Geometry check sheet. Reference: the model listing, model coordinates, mm. A direction names the side the tool comes from. Round coordinates to 2 decimals unless told otherwise and drop trailing zeros. Order: outer loops, then holes, each group sorted by start corner. A loop starts at its lowest first (then second) coordinate and runs counter-clockwise, first axis right, second up.
(1) Cross-section at B-B on x = 1.3. Count the separate pieces of the cut face and the enclosed holes in it, and give its area (3 significant figures).
(2) Cross-section at A-A on y = 105.5. Enter the section's corners in (x, z), and give its area (3 significant figures).
(3) Thickness scan on L1, parallel to Y at x = 0.95, z = 73.5; L2, parallel to Y at x = 1.4, z = 54; L3, parallel to Z at x = 0.15, y = -62.5. Record the ranges inside material, lowest first.
(4) Draft check along Y on faces 3 (the face through (0.811, -92.508, 55.896)), 4 (the face through (0.811, 154.312, 24.605)), 5 (the face through (0.789, 158.651, 69.018)). Enter one of: pulls with the +Y half, pulls with the -Y half, needs draft (parallel to the pull), parting line crosses it, or undercut.
(5) Cross-section at C-C on y = 177.5. Enter the section's corners in (x, z).
(6) Set-up check for faces 1 (the face through (1.6, 16, 38)), 2 (the face through (0.81, 139.3, 51.42)): record each of +Z, -Z, +X, -X, +Y, -Y from which the full face is reachable in a straight line by a thin tool's end or side.
(7) Gauge pin test, flat end, axial feed: P1, Ø3.5, axis at y = 189.88, z = 74, coming from the -X side. Record the tip position at first contact, or that the pin passes through.
Autodesk Inventor part; units mm, degrees
ref_plane "YZ Plane" through (0, 0, 0) normal (1, 0, 0) x (0, 1, 0)
ref_plane "XZ Plane" through (0, 0, 0) normal (0, 1, 0) x (-1, 0, 0)
ref_plane "XY Plane" through (0, 0, 0) normal (0, 0, 1) x (1, 0, 0)
sketch "Esquisse1" plane through (0, 0, 0) normal (1, 0, 0) x (0, 1, 0)
  line L0 (-80, -0.3825) -> (90, -0.3825)
  line L1 (90, -0.3825) -> (155.7273, 23)
  line L2 (155.7273, 23) -> (198, 78)
  line L3 (-80, -0.3825) -> (-102, 18)
  line L4 (-102, 18) -> (-95, 57)
  line L5 (-95, 57) -> (-53, 96)
  line L6 (-53, 96) -> (-9, 96)
  line L7 (-9, 96) -> (60.3686, 39.2438)
  line L8 (60.3686, 39.2438) -> (141.4545, 48)
  line L9 (141.4545, 48) -> (166, 78)
  line L10 (166, 78) -> (198, 78)
  point P0 (0, 0)
  dimension "d0" = 300
  dimension "d1" = 32
  dimension "d2" = 44
  dimension "d3" = 170
extrude "Extrusion1" add sketch "Esquisse1" along normal blind 1.6
fillet "Congé1" radius 50 6 edges at (0.8, -95, 57) (0.8, -80, -0.3825) (0.8, 60.3686, 39.2438) (0.8, 141.4545, 48) (0.8, 155.7273, 23) (0.8, 90, -0.3825)
fillet "Congé2" radius 10 1 edges at (0.8, -102, 18)
fillet "Congé3" radius 10 1 edges at (0.8, 166, 78)
fillet "Congé4" radius 2 1 edges at (0.8, 198, 78)
fillet "Congé5" radius 5 2 edges at (0.8, -9, 96) (0.8, -53, 96)
sketch "Esquisse2" plane through (1.6, 0, 0) normal (1, 0, 0) x (0, 0, -1)
  line L0 (-94.664, -54.4388) -> (-68.3658, -82.7599)
  arc A0 (-23.7165, -100.974) -> (-14.2761, -97.5432) centre (-21.9498, -91.1313) ccw
  line L1 (-14.2761, -97.5432) -> (-11.2486, -93.92)
  line L2 (0.3825, -61.8602) -> (0.3825, 81.3711)
  line L3 (-34.6945, 164.7156) -> (-74.7812, 195.5261)
  line L4 (-78, 193.9403) -> (-78, 170.7388)
  line L5 (-52.5054, 44.1601) -> (-94.8698, -7.6186)
  circle A1 centre (-89.1175, -53.974) radius 2
  circle A2 centre (-19.9498, -95.7558) radius 2
  circle A3 centre (-6.6175, -30.7558) radius 2
  circle A4 centre (-39, 10.1327) radius 2
  circle A5 centre (-20.5549, 80.7442) radius 2
  circle A6 centre (-45.9957, 155.7442) radius 2
  circle A7 centre (-6.6175, 29.2442) radius 2
  circle A8 centre (-74, 189.8806) radius 2
  line L6 (-40.5594, -97.9509) -> (-23.7165, -100.974)
  circle A9 centre (-52.9562, -87.598) radius 2
  circle A10 centre (-89.1175, -8.974) radius 2
  line L7 (-96, -10.7848) -> (-96, -51.0365)
  point P0 (-41.4923, 81.1901)
  point P1 (0, 0)
  dimension "d11" = 4
  dimension "d13" = 4
  dimension "d14" = 4
  dimension "d15" = 4
  dimension "d16" = 4
  dimension "d17" = 4
  dimension "d22" = 2
  dimension "d23" = 5.5
  dimension "d24" = 7
  dimension "d25" = 4
  dimension "d26" = 7
  dimension "d27" = 60
  dimension "d28" = 65
  dimension "d31" = 41.8748
  dimension "d32" = 20.9374
  dimension "d36" = 14
  dimension "d37" = 75
  dimension "d38" = 4
  dimension "d39" = 4
  dimension "d40" = 4
  dimension "d43" = 4
  dimension "d44" = 8
  dimension "d45" = 8
  dimension "d47" = 4
  dimension "d48" = 45
  dimension "d49" = 89.5
  dimension "d50" = 89.5
  dimension "d51" = 47
  dimension "d53" = 32
  dimension "d54" = 57
  dimension "d55" = 51.5
extrude "Extrusion2" cut sketch "Esquisse2" against normal blind 4
sketch "Esquisse4" plane through (1.6, 0, 0) normal (1, 0, 0) x (0, 0, -1)
  circle A0 centre (-20.5549, 80.7442) radius 2
  line L0 (-52.5054, 44.1601) -> (-94.8698, -7.6186)
  arc A1 (-47.0739, 50.7986) -> (-71.5553, 20.8768) centre (-55.3427, 32.5879) ccw
  line L1 (-47.0739, 50.7986) -> (-71.5553, 20.8768)
  point P0 (-96, -10.7848)
  point P1 (0, 0)
  dimension "d62" = 40
  dimension "d63" = 40
  dimension "d64" = 20
extrude "Extrusion4" add sketch "Esquisse4" against normal blind 1.6 contours L0 A1 L1
fillet "Congé7" radius 20 2 edges at (0.8, 20.8768, 71.5553) (0.8, 51.09, 47.7484)
sketch "Esquisse5" plane through (1.6, 0, 0) normal (1, 0, 0) x (0, 0, -1)
  line L0 (0.3825, -61.8602) -> (0.3825, 81.3711)
  circle A0 centre (-19.9498, -95.7558) radius 2
  circle A1 centre (-64.6175, 39.2442) radius 2
  point P0 (0, 0)
  dimension "d68" = 4
  dimension "d69" = 65
  dimension "d70" = 135
extrude "Extrusion5" cut sketch "Esquisse5" against normal through all contours A1
equation "\"d13\" = d11"
equation "\"d14\" = d11"
equation "\"d15\" = d11"
equation "\"d16\" = d11"
equation "\"d17\" = d11"
equation "\"d25\" = d11"
equation "\"d26\" = d24"
equation "\"d32\" = 0.5 * d31"
equation "\"d38\" = d11"
equation "\"d43\" = d11"
equation "\"d47\" = d11"
equation "\"d50\" = d49"
equation "\"d41\" = d43"
properties part number "Cote_Gauche" material "Fibre de verre - FR4"
Found:
1. separate pieces: 1
1. enclosed holes: 11
1. area: 17,300 mm2
2. outline: (0, 5.13) - (1.6, 5.13) - (1.6, 44.12) - (0, 44.12) - close
2. area: 62.4 mm2
3. L1: y = -77.23 to 40.97, 162.32 to 187.94, 191.82 to 194.54
3. L2: y = -93.5 to -89.3, -85.89 to 53.55, 143.6 to 179.55
3. L3: z = -0.38 to 87.18
4. face 3: pulls with the -Y half
4. face 4: pulls with the +Y half
4. face 5: undercut
5. outline: (0, 51.33) - (1.6, 51.33) - (1.6, 78) - (0, 78) - close
6. face 1: +Z, -Z, +X, +Y, -Y
6. face 2: +Z, +X, -X
7. P1: passes through
